from build123d import *

# Parameters (mm, degrees)
F0_W     = 700
F0_H     = 50
F1_DEPTH = 15
F2_W     = 110
F2_H     = 7.5
F3_DEPTH = 50.001
F5_D     = 3.3
F7_D     = 3.3
F9_D     = 7
F11_D    = 6.5


with BuildPart() as f1:
    # F0 (on Front) → F1 (new body)
    with BuildSketch(Plane.XZ):
        Rectangle(F0_W, F0_H)
    extrude(amount=F1_DEPTH)

    # F2 (on face) → F3 (cut, through all)
    with BuildSketch(Plane(origin=(0, 0, -25), x_dir=(1, 0, 0), z_dir=(0, 0, -1))):
        with Locations((295, 11.25)):
            Rectangle(F2_W, F2_H)
    extrude(amount=-F3_DEPTH, mode=Mode.SUBTRACT)

    # F5 (through all)
    with Locations(Plane(origin=(0, 0, 0), x_dir=(-1, 0, 0), z_dir=(0, 1, 0))):
        with Locations((-311.5, 0), (-278.5, 0)):
            Hole(F5_D / 2)

    # F7 (through all)
    with Locations(Plane(origin=(0, 0, 0), x_dir=(-1, 0, 0), z_dir=(0, 1, 0))):
        with Locations((312, 0), (345, 0)):
            Hole(F7_D / 2)

    # F9 (through all)
    with Locations(Plane(origin=(0, 0, 0), x_dir=(-1, 0, 0), z_dir=(0, 1, 0))):
        with Locations((-230, 0)):
            Hole(F9_D / 2)

    # F11 (through all)
    with Locations(Plane(origin=(0, 0, 0), x_dir=(-1, 0, 0), z_dir=(0, 1, 0))):
        with Locations((-345, 0), (-245, 0)):
            Hole(F11_D / 2)


solid = f1.part
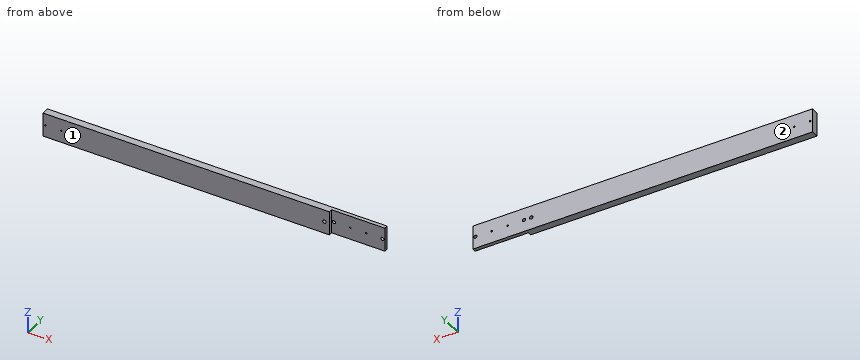
Build history of the part. All positions in model axes, mm. Face numbers are marked on the shaded views. Coordinates: 2 decimals unless noted, no trailing zeros. Order: outer loops, then holes, each group sorted by start corner. A loop starts at its lowest first (then second) coordinate and runs counter-clockwise, first axis right, second up. Notation, with made-up numbers: M 5,44 L 31,44 A26 cw 31,77 Z; hole C 80.25,37.5 d7. An arc over 180 degrees is marked long. One line per question, with ' | ' between items. Start each with the question number.
Q1. Saw through at B-B (z = -15). List the corners of the cut face in (x, y).
Q2. Saw through at A-A (y = -11). List the corners of the cut face in (x, z), then the cut area to 3 significant figures.
Q3. Two-plate mould, pull along Y, no slides. Class the marked faces 1 and 2: +Y half, -Y half, draft (parallel to the pull), parting line (faces both ways), or undercut.
Q4. Flat gauge pins, fed straight in: pin 1 Ø8.5 at (x, z) = (245, 0) entering from -Y; pin 2 Ø4 at (y, z) = (-11.5, -4) entering from +X. Where does each tip first touch, or does it go through?
Q5. Probe L1, parallel to Z at x = -345, y = -4.5; L2, parallel to Z at x = 230, y = -12; L3, parallel to Y at x = 284, z = 21. List the from-to ranges inside material, lowest first. Write a range as from..to.
Check values:
1) outline: M -350,-15 L 240,-15 L 240,-7.5 L 350,-7.5 L 350,0 L -350,0 Z
2) outline: M -350,-25 L 240,-25 L 240,25 L -350,25 Z; hole C -345,0 d3.3; hole C -312,0 d3.3; hole C 230,0 d7 | area: 29,400 mm2
3) face 1: -Y half | face 2: +Y half
4) pin 1: stops at y = -7.5 | pin 2: stops at x = 240
5) L1: z = -25..-1.65, 1.65..25 | L2: z = -25..-3.5, 3.5..25 | L3: y = -7.5..0
